```python
from build123d import *

# Parameters (mm, degrees)
F3_DEPTH  = 5.08
F6_DEPTH  = 5.08
F7_DEPTH  = 21.59
F8_R      = 7.8994
F9_DEPTH  = 25.4
F10_R     = 3.429
F11_DEPTH = 25.4
F12_R     = 2.667
F13_DEPTH = 25.4
F14_R     = 2.667
F15_DEPTH = 25.4
F1_R      = 1.4605
F16_DEPTH = 3.6068
F0_R      = 1.6129
F17_DEPTH = 3.6068
F18_R     = 1.905
F19_DEPTH = 12.7
F20_R     = 2
F21_DEPTH = 25.4


with BuildPart() as f3:
    # F2 (on Top) → F3 (new body)
    with BuildSketch(Plane.XY):
        Polygon((-43.589437, -12.7), (0, -12.7), (110.36633, -12.7), (110.36633, 85.2678), (0, 85.2678), (-43.589437, 85.2678), (-43.589437, 72.5678), (-43.589437, 0), align=None)
    extrude(amount=-F3_DEPTH)

    # F4 (on Top) → F6 (join)
    with BuildSketch(Plane.XY):
        Polygon((110.394933, 90.221972), (-5.796864, 90.221972), (-43.560833, 90.221972), (-48.640833, 90.221972), (-48.640833, 85.141972), (-48.640833, -12.825828), (-48.640833, -17.905828), (-43.560833, -17.905828), (-5.796864, -17.905828), (110.394933, -17.905828), (115.474933, -17.905828), (115.474933, -12.825828), (115.474933, 85.141972), (115.474933, 90.221972), align=None)
        Polygon((110.394933, -12.825828), (-5.796864, -12.825828), (-43.560833, -12.825828), (-43.560833, 85.141972), (-5.796864, 85.141972), (110.394933, 85.141972), align=None, mode=Mode.SUBTRACT)
    extrude(amount=-F6_DEPTH)

    # F5 (on face) → F7 (join)
    with BuildSketch(Plane.XY):
        Polygon((110.394933, 90.221972), (-5.796864, 90.221972), (-43.560833, 90.221972), (-48.640833, 90.221972), (-48.640833, 85.141972), (-48.640833, -12.825828), (-48.640833, -17.905828), (-43.560833, -17.905828), (-5.796864, -17.905828), (110.394933, -17.905828), (115.474933, -17.905828), (115.474933, 48.9839), (115.474933, 90.221972), align=None)
        Polygon((110.394933, -12.825828), (-5.796864, -12.825828), (-43.560833, -12.825828), (-43.560833, 85.141972), (-5.796864, 85.141972), (110.394933, 85.141972), align=None, mode=Mode.SUBTRACT)
    extrude(amount=F7_DEPTH)

    # F8 (on face) → F9 (cut)
    with BuildSketch(Plane(origin=(0, 90.221972, 0), x_dir=(-1, 0, 0), z_dir=(0, 1, 0))):
        with Locations((24.494825, 10.795)):
            Circle(F8_R)
    extrude(amount=-F9_DEPTH, mode=Mode.SUBTRACT)

    # F10 (on face) → F11 (cut)
    with BuildSketch(Plane(origin=(0, 90.221972, 0), x_dir=(-1, 0, 0), z_dir=(0, 1, 0))):
        with Locations((-90.13474, 10.795)):
            Circle(F10_R)
    extrude(amount=-F11_DEPTH, mode=Mode.SUBTRACT)

    # F12 (on face) → F13 (cut)
    with BuildSketch(Plane(origin=(-48.640833, 0, 0), x_dir=(0, -1, 0), z_dir=(-1, 0, 0))):
        with Locations((-21.966936, 10.795)):
            Circle(F12_R)
    extrude(amount=-F13_DEPTH, mode=Mode.SUBTRACT)

    # F14 (on face) → F15 (cut)
    with BuildSketch(Plane.YZ.offset(115.474933)):
        with Locations((37.101891, 10.795)):
            Circle(F14_R)
    extrude(amount=-F15_DEPTH, mode=Mode.SUBTRACT)

    # F1 (on Top) → F16 (cut)
    with BuildSketch(Plane.XY):
        with Locations((7.2644, 70.026379)):
            Circle(F1_R)
        with Locations((36.1696, 54.354579)):
            Circle(F1_R)
    extrude(amount=-F16_DEPTH, mode=Mode.SUBTRACT)

    # F0 (on Top) → F17 (cut)
    with BuildSketch(Plane.XY):
        with Locations((3.7592, 35.814)):
            Circle(F0_R)
        with Locations((3.7592, 5.969)):
            Circle(F0_R)
        with Locations((66.1162, 5.969)):
            Circle(F0_R)
        with Locations((66.1162, 35.814)):
            Circle(F0_R)
    extrude(amount=-F17_DEPTH, mode=Mode.SUBTRACT)

    # F18 (on face) → F19 (cut)
    with BuildSketch(Plane.XY.offset(21.59)):
        with Locations((-46.100833, -15.365828)):
            Circle(F18_R)
        with Locations((-46.100833, 87.681972)):
            Circle(F18_R)
        with Locations((112.934933, 87.681972)):
            Circle(F18_R)
        with Locations((112.934933, -15.365828)):
            Circle(F18_R)
    extrude(amount=-F19_DEPTH, mode=Mode.SUBTRACT)

    # F20 (on face) → F21 (cut)
    with BuildSketch(Plane.XY):
        with Locations((-25.017252, 36.220986)):
            Circle(F20_R)
        with Locations((91.822748, 36.220986)):
            Circle(F20_R)
    extrude(amount=-F21_DEPTH, mode=Mode.SUBTRACT)


solid = f3.part
```
Could you check a few things on this model? Use its own coordinates, in mm. A direction names the side the tool comes from. Round coordinates to 2 decimals unless told otherwise and drop trailing zeros. Loops run counter-clockwise (first coordinate to the right, second up) from the corner with the lowest first, then second, coordinate; pieces in that order, holes last. Notation, with made-up numbers: (37.5, 15) - (42.5, 15) arc R22 ccw to (42.5, 32) - close; hole circle Ø2 at (-18.5, 9.5). An arc over 180 degrees is marked (long way). Use CSV: the item, a comma, the result in double quotes.
Item 1: If we mould it in two halves opening along Z, with no side actions, what happens to faces 1 (the flat face through (4, 36, -3.607)), 2 (the cylindrical face through (-46.14, 24.63, 10.91)), 3 (the cylindrical face through (3.549, 37.413, -1.778))? For each: pulls with the +Z half, pulls with the -Z half, needs draft (parallel to the pull), parting line crosses it, or undercut.
Here are the results:
face 1,"pulls with the +Z half"
face 2,"undercut"
face 3,"needs draft"
Item 2: If we section it at D-D on x = -21: List the corners of the cut face in (y, z) for me.
Here are the results:
outline,"(-17.91, -5.08) - (-12.83, -5.08) - (-12.83, 21.59) - (-17.91, 21.59) - close; (-12.7, -5.08) - (90.22, -5.08) - (90.22, 3.71) - (85.14, 3.71) - (85.14, 0) - (-12.7, 0) - close; (85.14, 17.88) - (90.22, 17.88) - (90.22, 21.59) - (85.14, 21.59) - close"
Item 3: For faces 4 (the flat face through (34, -12.826, 8)), 5 (the flat face through (-48.641, 37, 8)), 6 (the flat face through (-46, -15, 8.89)), 7 (the cylindrical face through (-16.6, 87.7, 11.1)), which set-ups out of +Z, -Z, +X, -X, +Y, -Y let a thin tool reach every point of the face, with its end or its side?
Here are the results:
face 4,"+Z, -Z"
face 5,"+Z, -Z, -X, +Y, -Y"
face 6,"+Z"
face 7,"+Y"
Item 4: Will these pins go through, and if not, where does the flat tip stop? pin 1 (6 mm diameter, centred on x = 112.93, y = 87.68, fed in from +Z); pin 2 (2.5 mm diameter, centred on x = -46.1, y = 87.68, fed in from +Z); pin 3 (3.5 mm diameter, centred on x = 65.5, y = 5.5, fed in from +Z).
Here are the results:
pin 1,"stops at z = 21.59"
pin 2,"stops at z = 8.89"
pin 3,"stops at z = 0"
Item 5: If we section it at A-A on y = 28.5: List the corners of the cut face in (x, z) for me.
Here are the results:
outline,"(-48.64, -5.08) - (110.37, -5.08) - (110.37, 0) - (-43.56, 0) - (-43.56, 21.59) - (-48.64, 21.59) - close; (110.39, -5.08) - (115.47, -5.08) - (115.47, 21.59) - (110.39, 21.59) - close"
Item 6: If we section it at C-C on z = 16.5: List the corners of the cut face in (x, y) for me (3 decimals), then the cut area to 3 significant figures.
Here are the results:
outline,"(-48.641, -17.906) - (115.475, -17.906) - (115.475, 90.222) - (-19.031, 90.222) - (-19.031, 85.142) - (110.395, 85.142) - (110.395, -12.826) - (-43.561, -12.826) - (-43.561, 85.142) - (-29.959, 85.142) - (-29.959, 90.222) - (-48.641, 90.222) - close; hole circle Ø3.81 at (-46.101, -15.366); hole circle Ø3.81 at (-46.101, 87.682); hole circle Ø3.81 at (112.935, -15.366); hole circle Ø3.81 at (112.935, 87.682)"
area,"2,560 mm²"
Item 7: If we section it at B-B on x = 22: List the corners of the cut face in (y, z) for me, then the cut area to 3 significant figures.
Here are the results:
outline,"(-17.91, -5.08) - (-12.83, -5.08) - (-12.83, 21.59) - (-17.91, 21.59) - close; (-12.7, -5.08) - (90.22, -5.08) - (90.22, 21.59) - (85.14, 21.59) - (85.14, 0) - (-12.7, 0) - close"
area,"768 mm²"
Item 8: I need wall thicknesses on L1, parallel to Y at x = 5.5, z = 4; L2, parallel to X at y = 15.5, z = 19.5; L3, parallel to Z at x = 25, y = 1.5. Which ranges of each line are inside material? Lowest first, please. Write a range as [from, to].
Here are the results:
L1,"y = [-17.91, -12.83], [85.14, 90.22]"
L2,"x = [-48.64, -43.56], [110.39, 115.47]"
L3,"z = [-5.08, 0]"
